```python
from build123d import *

# Parameters (mm, degrees)
SKETCH1_R           = 2.5
BOSS_EXTRUDE1_DEPTH = 1.7
CUT_EXTRUDE4_DEPTH  = 24.372045268
SKETCH6_W           = 17.56
SKETCH6_H           = 1.7
BOSS_EXTRUDE4_DEPTH = 7.5
SKETCH9_W           = 8
SKETCH9_H           = 2
CUT_EXTRUDE2_DEPTH  = 0.7
FILLET1_R           = 1


with BuildPart() as part:
    # Sketch1 → Boss-Extrude1 (new body)
    with BuildSketch(Plane.XY):
        with BuildLine():
            Line((0, 0), (17.56, 0))
            Line((17.56, 0), (17.56, 6.55))
            ThreePointArc((17.56, 6.55), (8.78, 15.33), (0, 6.55))
            Line((0, 6.55), (0, 0))
        make_face()
        with Locations((8.78, 8.5)):
            Circle(SKETCH1_R, mode=Mode.SUBTRACT)
    extrude(amount=BOSS_EXTRUDE1_DEPTH)

    # Sketch3 → Cut-Extrude4 (cut, through all)
    with BuildSketch(Plane.XY.offset(1.7)):
        with BuildLine():
            ThreePointArc((12.24, 14.619498126), (8.78, 15.33), (5.32, 14.619498126))
            Line((5.32, 14.619498126), (12.24, 14.619498126))
        make_face()
    extrude(amount=-CUT_EXTRUDE4_DEPTH, mode=Mode.SUBTRACT)

    # Sketch6 → Boss-Extrude4 (add)
    with BuildSketch(Plane.XZ):
        with Locations((8.78, 0.85)):
            Rectangle(SKETCH6_W, SKETCH6_H)
    extrude(amount=BOSS_EXTRUDE4_DEPTH)

    # Sketch9 → Cut-Extrude2 (cut)
    with BuildSketch(Plane.XY.offset(1.7)):
        with Locations((8.78, -5.353166831)):
            Rectangle(SKETCH9_W, SKETCH9_H)
    extrude(amount=-CUT_EXTRUDE2_DEPTH, mode=Mode.SUBTRACT)

    # Fillet1
    # the kernel refuses this fillet: 1 mm, written as the material it takes off along each edge
    with BuildSketch(Plane(origin=(12.78, -4.353166831, 1.7), x_dir=(1, 0, 0), z_dir=(0, -1, 0)), Plane(origin=(4.78, -6.353166831, 1.7), x_dir=(-1, 0, 0), z_dir=(0, 1, 0))) as fillet1_piece_1:
        with BuildLine():
            CenterArc((0.953939201, -1), FILLET1_R, 90, 72.542396876)
            Line((0, -0.7), (-0.019078784, -0.694))
            ThreePointArc((-0.019078784, -0.694), (-0.02, -0.35), (-0.02, 0))
            Line((-0.02, 0), (0, 0.02))
            Line((0, 0.02), (0.953939201, 0.02))
            Line((0.953939201, 0.02), (0.953939201, 0))
        make_face()
    extrude(amount=2, mode=Mode.SUBTRACT)
    with BuildSketch(Plane(origin=(12.78, -6.353166831, 1.7), x_dir=(0, -1, 0), z_dir=(-1, 0, 0)), Plane(origin=(4.78, -4.353166831, 1.7), x_dir=(0, 1, 0), z_dir=(1, 0, 0))) as fillet1_piece_2:
        with BuildLine():
            CenterArc((0.953939201, -1), FILLET1_R, 90, 72.542396876)
            Line((0, -0.7), (-0.019078784, -0.694))
            ThreePointArc((-0.019078784, -0.694), (-0.02, -0.35), (-0.02, 0))
            Line((-0.02, 0), (0, 0.02))
            Line((0, 0.02), (0.953939201, 0.02))
            Line((0.953939201, 0.02), (0.953939201, 0))
        make_face()
    extrude(amount=8, mode=Mode.SUBTRACT)
    with BuildSketch(Plane(origin=(12.78, -1.968318828, 1.7), x_dir=(1, 0, 0), z_dir=(0, -1, 0))) as fillet1_piece_3a_section:
        with BuildLine():
            CenterArc((0.953939201, -1), FILLET1_R, 90, 72.542396876)
            Line((0, -0.7), (-0.019078784, -0.694))
            ThreePointArc((-0.019078784, -0.694), (-0.02, -0.35), (-0.02, 0))
            Line((-0.02, 0), (0, 0.02))
            Line((0, 0.02), (0.953939201, 0.02))
            Line((0.953939201, 0.02), (0.953939201, 0))
        make_face()
    fillet1_piece_3a = extrude(amount=4.384848004, mode=Mode.PRIVATE)
    fillet1_piece_3a = split(fillet1_piece_3a, bisect_by=Plane(origin=(13.007122588, -4.353166831, 1.5212182), z_dir=(0, 1, 0)), keep=Keep.TOP, mode=Mode.PRIVATE)
    with BuildSketch(Plane(origin=(4.78, -4.353166831, 1.7), x_dir=(0, 1, 0), z_dir=(1, 0, 0))) as fillet1_piece_3b_section:
        with BuildLine():
            CenterArc((0.953939201, -1), FILLET1_R, 90, 72.542396876)
            Line((0, -0.7), (-0.019078784, -0.694))
            ThreePointArc((-0.019078784, -0.694), (-0.02, -0.35), (-0.02, 0))
            Line((-0.02, 0), (0, 0.02))
            Line((0, 0.02), (0.953939201, 0.02))
            Line((0.953939201, 0.02), (0.953939201, 0))
        make_face()
    fillet1_piece_3b = extrude(amount=10.384848004, mode=Mode.PRIVATE)
    fillet1_piece_3b = split(fillet1_piece_3b, bisect_by=Plane(origin=(12.78, -4.126044244, 1.5212182), z_dir=(1, 0, 0)), keep=Keep.TOP, mode=Mode.PRIVATE)
    fillet1_piece_3 = fillet1_piece_3a & fillet1_piece_3b
    add(fillet1_piece_3, mode=Mode.SUBTRACT)
    with BuildSketch(Plane(origin=(12.78, -4.353166831, 1.7), x_dir=(1, 0, 0), z_dir=(0, -1, 0))) as fillet1_piece_4a_section:
        with BuildLine():
            CenterArc((0.953939201, -1), FILLET1_R, 90, 72.542396876)
            Line((0, -0.7), (-0.019078784, -0.694))
            ThreePointArc((-0.019078784, -0.694), (-0.02, -0.35), (-0.02, 0))
            Line((-0.02, 0), (0, 0.02))
            Line((0, 0.02), (0.953939201, 0.02))
            Line((0.953939201, 0.02), (0.953939201, 0))
        make_face()
    fillet1_piece_4a = extrude(amount=4.384848004, mode=Mode.PRIVATE)
    fillet1_piece_4a = split(fillet1_piece_4a, bisect_by=Plane(origin=(13.007122588, -6.353166831, 1.5212182), z_dir=(0, -1, 0)), keep=Keep.TOP, mode=Mode.PRIVATE)
    with BuildSketch(Plane(origin=(15.164848004, -6.353166831, 1.7), x_dir=(0, -1, 0), z_dir=(-1, 0, 0))) as fillet1_piece_4b_section:
        with BuildLine():
            CenterArc((0.953939201, -1), FILLET1_R, 90, 72.542396876)
            Line((0, -0.7), (-0.019078784, -0.694))
            ThreePointArc((-0.019078784, -0.694), (-0.02, -0.35), (-0.02, 0))
            Line((-0.02, 0), (0, 0.02))
            Line((0, 0.02), (0.953939201, 0.02))
            Line((0.953939201, 0.02), (0.953939201, 0))
        make_face()
    fillet1_piece_4b = extrude(amount=10.384848004, mode=Mode.PRIVATE)
    fillet1_piece_4b = split(fillet1_piece_4b, bisect_by=Plane(origin=(12.78, -6.580289419, 1.5212182), z_dir=(1, 0, 0)), keep=Keep.TOP, mode=Mode.PRIVATE)
    fillet1_piece_4 = fillet1_piece_4a & fillet1_piece_4b
    add(fillet1_piece_4, mode=Mode.SUBTRACT)
    with BuildSketch(Plane(origin=(4.78, -8.738014835, 1.7), x_dir=(-1, 0, 0), z_dir=(0, 1, 0))) as fillet1_piece_5a_section:
        with BuildLine():
            CenterArc((0.953939201, -1), FILLET1_R, 90, 72.542396876)
            Line((0, -0.7), (-0.019078784, -0.694))
            ThreePointArc((-0.019078784, -0.694), (-0.02, -0.35), (-0.02, 0))
            Line((-0.02, 0), (0, 0.02))
            Line((0, 0.02), (0.953939201, 0.02))
            Line((0.953939201, 0.02), (0.953939201, 0))
        make_face()
    fillet1_piece_5a = extrude(amount=4.384848004, mode=Mode.PRIVATE)
    fillet1_piece_5a = split(fillet1_piece_5a, bisect_by=Plane(origin=(4.552877412, -6.353166831, 1.5212182), z_dir=(0, -1, 0)), keep=Keep.TOP, mode=Mode.PRIVATE)
    with BuildSketch(Plane(origin=(12.78, -6.353166831, 1.7), x_dir=(0, -1, 0), z_dir=(-1, 0, 0))) as fillet1_piece_5b_section:
        with BuildLine():
            CenterArc((0.953939201, -1), FILLET1_R, 90, 72.542396876)
            Line((0, -0.7), (-0.019078784, -0.694))
            ThreePointArc((-0.019078784, -0.694), (-0.02, -0.35), (-0.02, 0))
            Line((-0.02, 0), (0, 0.02))
            Line((0, 0.02), (0.953939201, 0.02))
            Line((0.953939201, 0.02), (0.953939201, 0))
        make_face()
    fillet1_piece_5b = extrude(amount=10.384848004, mode=Mode.PRIVATE)
    fillet1_piece_5b = split(fillet1_piece_5b, bisect_by=Plane(origin=(4.78, -6.580289419, 1.5212182), z_dir=(-1, 0, 0)), keep=Keep.TOP, mode=Mode.PRIVATE)
    fillet1_piece_5 = fillet1_piece_5a & fillet1_piece_5b
    add(fillet1_piece_5, mode=Mode.SUBTRACT)
    with BuildSketch(Plane(origin=(2.395151996, -4.353166831, 1.7), x_dir=(0, 1, 0), z_dir=(1, 0, 0))) as fillet1_piece_6a_section:
        with BuildLine():
            CenterArc((0.953939201, -1), FILLET1_R, 90, 72.542396876)
            Line((0, -0.7), (-0.019078784, -0.694))
            ThreePointArc((-0.019078784, -0.694), (-0.02, -0.35), (-0.02, 0))
            Line((-0.02, 0), (0, 0.02))
            Line((0, 0.02), (0.953939201, 0.02))
            Line((0.953939201, 0.02), (0.953939201, 0))
        make_face()
    fillet1_piece_6a = extrude(amount=10.384848004, mode=Mode.PRIVATE)
    fillet1_piece_6a = split(fillet1_piece_6a, bisect_by=Plane(origin=(4.78, -4.126044244, 1.5212182), z_dir=(-1, 0, 0)), keep=Keep.TOP, mode=Mode.PRIVATE)
    with BuildSketch(Plane(origin=(4.78, -6.353166831, 1.7), x_dir=(-1, 0, 0), z_dir=(0, 1, 0))) as fillet1_piece_6b_section:
        with BuildLine():
            CenterArc((0.953939201, -1), FILLET1_R, 90, 72.542396876)
            Line((0, -0.7), (-0.019078784, -0.694))
            ThreePointArc((-0.019078784, -0.694), (-0.02, -0.35), (-0.02, 0))
            Line((-0.02, 0), (0, 0.02))
            Line((0, 0.02), (0.953939201, 0.02))
            Line((0.953939201, 0.02), (0.953939201, 0))
        make_face()
    fillet1_piece_6b = extrude(amount=4.384848004, mode=Mode.PRIVATE)
    fillet1_piece_6b = split(fillet1_piece_6b, bisect_by=Plane(origin=(4.552877412, -4.353166831, 1.5212182), z_dir=(0, 1, 0)), keep=Keep.TOP, mode=Mode.PRIVATE)
    fillet1_piece_6 = fillet1_piece_6a & fillet1_piece_6b
    add(fillet1_piece_6, mode=Mode.SUBTRACT)


solid = part.part
```
The listing builds one solid part. Answer for the finished solid, in the listing's coordinates (mm). A direction names the side the tool comes from. Coordinates: 2 decimals unless noted, no trailing zeros. Write each loop counter-clockwise with the first axis right and the second up, starting at its lowest first coordinate (ties: lowest second). Pieces come first, ordered by that corner, then holes. Notation, with made-up numbers: (47.25, -4) - (58.25, -4) arc R31 ccw to (58.25, 25) - close; hole circle Ø10 at (89, 21.5). An arc over 180 degrees is marked (long way). Return JSON: item names as keys, results as strings. Group by question number.
Q1. Find the intervals of material crossed by line 1 along Y through (x, z) = (8.78, 0.4); line 2 along Y through (x, z) = (11, 1.15); line 3 along Y through (x, z) = (8.5, 1.55), in increasing order. Write a range as [from, to].
Q2. The part is cut by section B-B on z = 0.75. Write down the section's boundary in (x, y), and give its area (3 significant figures).
Q3. Which of the six approach directions +Z, -Z, +X, -X, +Y, -Y give full straight-line access (tool end or side, diameter ignored) to faces 1 (the cylindrical face through (4.291, -5.381, 1.585)), 2 (the cylindrical face through (1.49, 11.44, 0.84))?
Q4. The part is cut by section A-A on x = 8.78. Write down the section's boundary in (y, z), and give its area (3 significant figures).
Q5. The part is cut by section C-C on y = 9.75. Write down the section's boundary in (x, z), and give its area (3 significant figures).
Q6. For a pull along Y with two mould halves and no side action, classify faces 3 (the flat face through (9, 4, 0)), 4 (the cylindrical face through (8.85, -6.72, 1.51)), 5 (the cylindrical face through (8.7, -4, 1.5)), 6 (the flat face through (9, -7.5, 1)) as +Y half, -Y half, draft (parallel to the pull), parting line (faces both ways), or undercut.
Q7. The part is cut by section D-D on x = 6. Write down the section's boundary in (y, z).
Q8. Flat-ended cylindrical pins translate along their axes: pin 1 Ø1.6 at (x, y) = (8.5, -6) entering from +Z; pin 2 Ø4 at (x, y) = (6, -2.5) entering from -Z; pin 3 Ø4 at (x, y) = (8.78, 8.5) entering from -Z. Find the tip coordinate at first contact, or state that the pin passes through.
Evaluation:
{
 "1": {"line 1": "y = [-7.5, 6], [11, 14.62]", "line 2": "y = [-7.5, -6.41], [-4.29, 7.35], [9.65, 14.62]", "line 3": "y = [-7.5, -6.78], [-3.93, 6.02], [10.98, 14.62]"},
 "2": {"outline": "(0, -7.5) - (17.56, -7.5) - (17.56, 6.55) arc R8.78 ccw to (12.24, 14.62) - (5.32, 14.62) arc R8.78 ccw to (0, 6.55) - close; hole circle Ø5 at (8.78, 8.5)", "area": "345 mm2"},
 "3": {"face 1": "+Z", "face 2": "+Z, -Z, -X, +Y"},
 "4": {"outline": "(-7.5, 0) - (6, 0) - (6, 1.7) - (-3.4, 1.7) arc R1 ccw to (-4.35, 1) - (-6.35, 1) arc R1 ccw to (-7.31, 1.7) - (-7.5, 1.7) - close; (11, 0) - (14.62, 0) - (14.62, 1.7) - (11, 1.7) - close", "area": "27.3 mm2"},
 "5": {"outline": "(0.6, 0) - (6.61, 0) - (6.61, 1.7) - (0.6, 1.7) - close; (10.95, 0) - (16.96, 0) - (16.96, 1.7) - (10.95, 1.7) - close", "area": "20.4 mm2"},
 "6": {"face 3": "draft", "face 4": "undercut", "face 5": "undercut", "face 6": "-Y half"},
 "7": {"outline": "(-7.5, 0) - (14.62, 0) - (14.62, 1.7) - (-3.4, 1.7) arc R1 ccw to (-4.35, 1) - (-6.35, 1) arc R1 ccw to (-7.31, 1.7) - (-7.5, 1.7) - close"},
 "8": {"pin 1": "stops at z = 1.56", "pin 2": "stops at z = 0", "pin 3": "passes through"}
}
